```python
from build123d import *

# Parameters (mm, degrees)
PCB_W           = 60
PCB_H           = 50
PCB_DEPTH       = 1.6
HOLE_0_R        = 1.5
HOLE_0_DEPTH    = 5
HOLE_1_R        = 1.5
HOLE_1_DEPTH    = 5
HOLE_2_R        = 1.5
HOLE_2_DEPTH    = 5
HOLE_3_R        = 1.5
HOLE_3_DEPTH    = 5
FLOOR_CUT_W     = 44.76
FLOOR_CUT_H     = 34.76
FLOOR_CUT_DEPTH = 1
BLOCK_0_W       = 8.62
BLOCK_0_H       = 8.62
BLOCK_0_DEPTH   = 5
BLOCK_1_W       = 8.62
BLOCK_1_H       = 8.62
BLOCK_1_DEPTH   = 5
BLOCK_2_W       = 8.62
BLOCK_2_H       = 8.62
BLOCK_2_DEPTH   = 5
BLOCK_3_W       = 8.62
BLOCK_3_H       = 8.62
BLOCK_3_DEPTH   = 5
FLOOR_W         = 62
FLOOR_H         = 52
FLOOR_DEPTH     = 1


with BuildPart() as pcb:
    # pcb → pcb (new body)
    with BuildSketch(Plane(origin=(1, 1, 3.4), x_dir=(1, 0, 0), z_dir=(0, 0, 1))):
        with Locations((30, 25)):
            Rectangle(PCB_W, PCB_H)
    extrude(amount=PCB_DEPTH)


with BuildPart() as hole_0_body:
    # hole_0 → hole_0 (new body)
    with BuildSketch(Plane(origin=(4.81, 4.81, 0), x_dir=(1, 0, 0), z_dir=(0, 0, 1))):
        Circle(HOLE_0_R)
    extrude(amount=HOLE_0_DEPTH)


with BuildPart() as hole_1_body:
    # hole_1 → hole_1 (new body)
    with BuildSketch(Plane(origin=(4.81, 47.19, 0), x_dir=(1, 0, 0), z_dir=(0, 0, 1))):
        Circle(HOLE_1_R)
    extrude(amount=HOLE_1_DEPTH)


with BuildPart() as hole_2_body:
    # hole_2 → hole_2 (new body)
    with BuildSketch(Plane(origin=(57.19, 4.81, 0), x_dir=(1, 0, 0), z_dir=(0, 0, 1))):
        Circle(HOLE_2_R)
    extrude(amount=HOLE_2_DEPTH)


with BuildPart() as hole_3_body:
    # hole_3 → hole_3 (new body)
    with BuildSketch(Plane(origin=(57.19, 47.19, 0), x_dir=(1, 0, 0), z_dir=(0, 0, 1))):
        Circle(HOLE_3_R)
    extrude(amount=HOLE_3_DEPTH)


with BuildPart() as tool:
    # floor_cut → floor_cut (new body)
    with BuildSketch(Plane(origin=(8.62, 8.62, 0), x_dir=(1, 0, 0), z_dir=(0, 0, 1))):
        with Locations((22.38, 17.38)):
            Rectangle(FLOOR_CUT_W, FLOOR_CUT_H)
    extrude(amount=FLOOR_CUT_DEPTH)

    # tool: union pcb, hole_0 body, hole_1 body, hole_2 body, hole_3 body
    add(pcb.part)
    add(hole_0_body.part)
    add(hole_1_body.part)
    add(hole_2_body.part)
    add(hole_3_body.part)


with BuildPart() as block_0_body:
    # block_0 → block_0 (new body)
    with BuildSketch(Plane.XY):
        with Locations((4.31, 4.31)):
            Rectangle(BLOCK_0_W, BLOCK_0_H)
    extrude(amount=BLOCK_0_DEPTH)


with BuildPart() as block_1_body:
    # block_1 → block_1 (new body)
    with BuildSketch(Plane(origin=(0, 43.38, 0), x_dir=(1, 0, 0), z_dir=(0, 0, 1))):
        with Locations((4.31, 4.31)):
            Rectangle(BLOCK_1_W, BLOCK_1_H)
    extrude(amount=BLOCK_1_DEPTH)


with BuildPart() as block_2_body:
    # block_2 → block_2 (new body)
    with BuildSketch(Plane(origin=(53.38, 0, 0), x_dir=(1, 0, 0), z_dir=(0, 0, 1))):
        with Locations((4.31, 4.31)):
            Rectangle(BLOCK_2_W, BLOCK_2_H)
    extrude(amount=BLOCK_2_DEPTH)


with BuildPart() as block_3_body:
    # block_3 → block_3 (new body)
    with BuildSketch(Plane(origin=(53.38, 43.38, 0), x_dir=(1, 0, 0), z_dir=(0, 0, 1))):
        with Locations((4.31, 4.31)):
            Rectangle(BLOCK_3_W, BLOCK_3_H)
    extrude(amount=BLOCK_3_DEPTH)


with BuildPart() as final:
    # floor → floor (new body)
    with BuildSketch(Plane.XY):
        with Locations((31, 26)):
            Rectangle(FLOOR_W, FLOOR_H)
    extrude(amount=FLOOR_DEPTH)

    # base: union block_0 body, block_1 body, block_2 body, block_3 body
    add(block_0_body.part)
    add(block_1_body.part)
    add(block_2_body.part)
    add(block_3_body.part)

    # final: cut tool
    add(tool.part, mode=Mode.SUBTRACT)


solid = final.part
```
Geometry check sheet. Reference: the model listing, model coordinates, mm. A direction names the side the tool comes from. Round coordinates to 2 decimals unless told otherwise and drop trailing zeros. Write each loop counter-clockwise with the first axis right and the second up, starting at its lowest first coordinate (ties: lowest second). Pieces come first, ordered by that corner, then holes. Notation, with made-up numbers: (31.5, 29.25) - (44.5, 29.25) arc R29 ccw to (44.5, 66.25) - close; hole circle Ø10 at (5, 45). An arc over 180 degrees is marked (long way). Write each question's results on one line, items separated by ' | '.
(1) Depth check by flat-ended pin: pin 1 Ø3.5 at (x, y) = (4.81, 47.19) entering from +Z; pin 2 Ø7 at (x, y) = (59.5, 24.5) entering from +Z. Enter the tip coordinate at first touch or a pass-through.
Computed:
pin 1: stops at z = 3.4 | pin 2: stops at z = 1
(2) Sectioned sample at B-B, the plane y = 26.5. Enter the section's corners in (x, z), plus the area to 3 significant figures.
Computed:
outline: (0, 0) - (8.62, 0) - (8.62, 1) - (0, 1) - close; (53.38, 0) - (62, 0) - (62, 1) - (53.38, 1) - close | area: 17.2 mm^2
(3) Thickness scan on probe 1 along Y at (x, z) = (4.81, 2.25); probe 2 along Y at (x, z) = (57.19, 0.8); probe 3 along X at (y, z) = (47.19, 0.75). Record the ranges inside material, lowest first. Write a range as from..to.
Computed:
probe 1: y = 0..3.31, 6.31..8.62, 43.38..45.69, 48.69..52 | probe 2: y = 0..3.31, 6.31..45.69, 48.69..52 | probe 3: x = 0..3.31, 6.31..55.69, 58.69..62
(4) Draft check along X on faces 1 (the face through (58, 26, 1)), 2 (the face through (31, 48, 1)), 3 (the face through (0, 19.9, 0.8)). Enter one of: pulls with the +X half, pulls with the -X half, needs draft (parallel to the pull), parting line crosses it, or undercut.
Computed:
face 1: needs draft | face 2: undercut | face 3: pulls with the -X half
(5) Sectioned sample at C-C, the plane y = 47.19. Enter the section's corners in (x, z), plus the area to 3 significant figures.
Computed:
outline: (0, 0) - (3.31, 0) - (3.31, 3.4) - (1, 3.4) - (1, 5) - (0, 5) - close; (6.31, 0) - (55.69, 0) - (55.69, 3.4) - (53.38, 3.4) - (53.38, 1) - (8.62, 1) - (8.62, 3.4) - (6.31, 3.4) - close; (58.69, 0) - (62, 0) - (62, 5) - (61, 5) - (61, 3.4) - (58.69, 3.4) - close | area: 86.2 mm^2
(6) Sectioned sample at A-A, the plane z = 1.8. Enter the section's corners in (x, y).
Computed:
outline: (0, 0) - (8.62, 0) - (8.62, 8.62) - (0, 8.62) - close; (0, 43.38) - (8.62, 43.38) - (8.62, 52) - (0, 52) - close; (53.38, 0) - (62, 0) - (62, 8.62) - (53.38, 8.62) - close; (53.38, 43.38) - (62, 43.38) - (62, 52) - (53.38, 52) - close; hole circle Ø3 at (4.81, 4.81); hole circle Ø3 at (4.81, 47.19); hole circle Ø3 at (57.19, 4.81); hole circle Ø3 at (57.19, 47.19)
(7) Set-up check for faces 4 (the face through (53.38, 48, 2)), 5 (the face through (2.4, 0.8, 5)), 6 (the face through (57, 51, 4)): record each of +Z, -Z, +X, -X, +Y, -Y from which the full face is reachable in a straight line by a thin tool's end or side.
Computed:
face 4: +Z, +Y, -Y | face 5: +Z, +X, -X, +Y, -Y | face 6: +Z
(8) Sectioned sample at D-D, the plane x = 40.5. Enter the section's corners in (y, z), plus the area to 3 significant figures.
Computed:
outline: (0, 0) - (8.62, 0) - (8.62, 1) - (0, 1) - close; (43.38, 0) - (52, 0) - (52, 1) - (43.38, 1) - close | area: 17.2 mm^2
